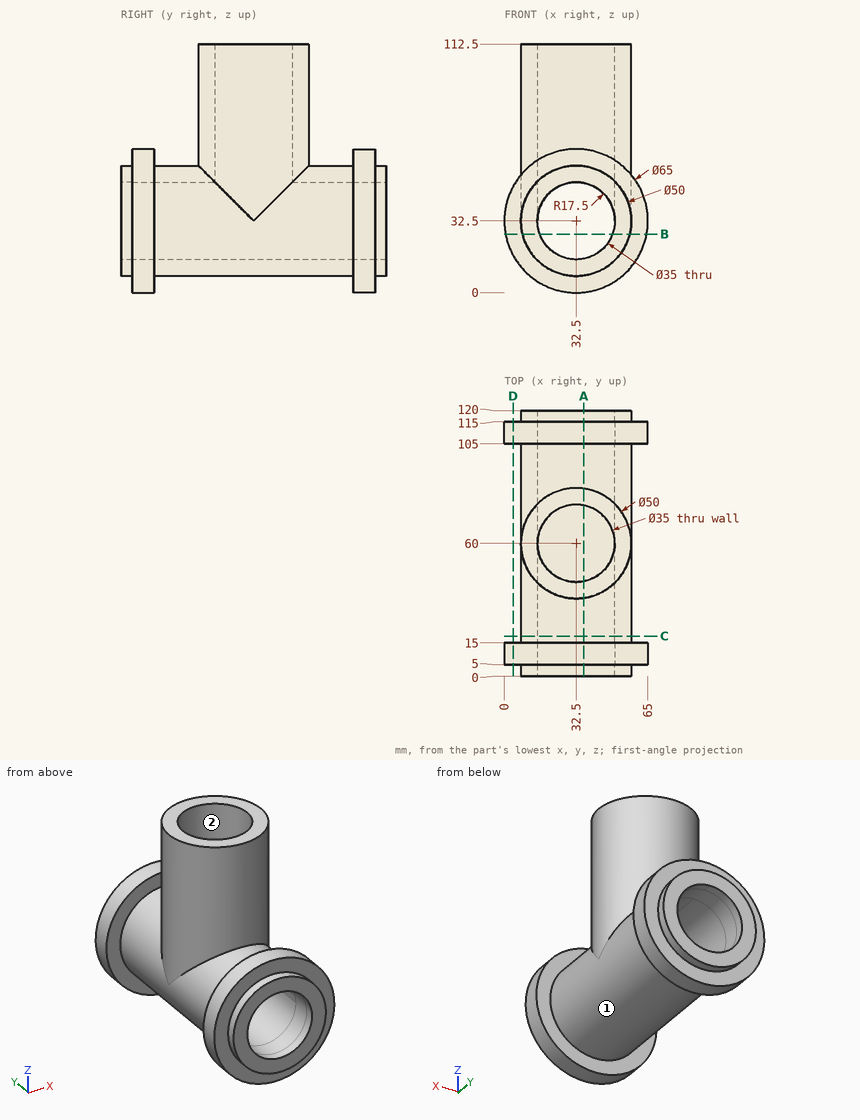
Could you check a few things on this drawing? It's one solid part, dimensions in mm from its lowest x, y, z. Give positions to 0.01 mm unless a question says otherwise; leave off trailing zeros. Loops run counter-clockwise (first coordinate to the right, second up) from the corner with the lowest first, then second, coordinate; pieces in that order, holes last. Notation, with made-up numbers: M 13.25,9 L 45.25,9 A22 cw 45.25,32 Z; hole C 34,-36.75 d3. An arc over 180 degrees is marked long. Answer as a JSON object with one key per item and string values.
Q1. Suppose I cut it at A-A, the plane x = 36. State how many separate pieces and enclosed holes the cut face has, plus the area to 3 significant figures.
Values found:
{"separate pieces": "3", "enclosed holes": "0", "area": "2,710 mm²"}
Q2. If I drill on probe 1 along X at (y, z) = (111, 32); probe 2 along X at (y, z) = (2, 32) (3 decimals); probe 3 along Y at (x, z) = (51, 9), over which ranges is the centre line in solid material (lowest first)? Write a range as [from, to].
Values found:
{"probe 1": "x = [0, 15.01], [49.99, 65]", "probe 2": "x = [7.505, 15.007], [49.993, 57.495]", "probe 3": "y = [5, 15], [105, 115]"}
Q3. Suppose I cut it at D-D, the plane x = 4. List the corners of the cut face in (y, z) for me, plus the area to 3 significant figures.
Values found:
{"outline": "M 5,16.88 L 15,16.88 L 15,48.12 L 5,48.12 Z; M 105,16.88 L 115,16.88 L 115,48.12 L 105,48.12 Z", "area": "625 mm²"}
Q4. Suppose I cut it at C-C, the plane y = 18. List the corners of the cut face in (x, z) for me, plus the area to 3 significant figures.
Values found:
{"outline": "C 32.5,32.5 d50; hole C 32.5,32.5 d35", "area": "1,000 mm²"}
Q5. If we mould it in two halves opening along X, with no side actions, what happens to the marked faces 1 and 2? For each: pulls with the +X half, pulls with the -X half, needs draft (parallel to the pull), parting line crosses it, or undercut.
Values found:
{"face 1": "parting line crosses it", "face 2": "undercut"}
Q6. For P1, Ø8, axis at x = 45, y = 87, coming from the -Z side; P2, Ø12, axis at x = 11, y = 95, coming from the +Z side; P3, Ø1, axis at y = 59.5, z = 61.5, coming from the -X side; P4, Ø21, axis at x = 32.5, z = 32.5, coming from the +Y side, each with a flat end and sliding along its axis, tell me the tip position at first contact or that it passes through.
Values found:
{"P1": "stops at z = 8.99", "P2": "stops at z = 52.12", "P3": "stops at x = 7.5", "P4": "passes through"}
Q7. Suppose I cut it at B-B, the plane z = 26.5. List the corners of the cut face in (x, y) for me, plus the area to 3 significant figures.
Values found:
{"outline": "M 0.56,5 L 8.23,5 L 8.23,0 L 16.06,0 L 16.06,120 L 8.23,120 L 8.23,115 L 0.56,115 L 0.56,105 L 8.23,105 L 8.23,15 L 0.56,15 Z; M 48.94,0 L 56.77,0 L 56.77,5 L 64.44,5 L 64.44,15 L 56.77,15 L 56.77,105 L 64.44,105 L 64.44,115 L 56.77,115 L 56.77,120 L 48.94,120 Z", "area": "2,190 mm²"}
